Here's how the part is built. I have some questions about the finished solid (model axes, mm). A direction names the side the tool comes from. Give positions to 0.01 mm unless a question says otherwise; leave off trailing zeros. Write each loop counter-clockwise with the first axis right and the second up, starting at its lowest first coordinate (ties: lowest second). Pieces come first, ordered by that corner, then holes. Notation, with made-up numbers: (41, -9.5) - (70, -9.5) arc R25 cw to (70, 11.5) - close; hole circle Ø6 at (14.5, 14.25). An arc over 180 degrees is marked (long way). One line per item, written item: value. Start each with the question number.
1) Please list where these lines run through material, in increasing order: L1, parallel to X at y = 1.45, z = 7.4; L2, parallel to X at y = 3.6, z = -4; L3, parallel to Z at x = 3, y = 0.55. Write a range as [from, to].
2) I'm going to push flat-ended pins straight in: P1, Ø3, axis at x = -17.9, z = -5.4, coming from the +Y side; P2, Ø1.8, axis at x = -13, z = 41.02, coming from the +Y side. Where does each tip first touch, or does it pass through?
3) We'd pull the mould along Z, two halves only. Please class faces 4 (the flat face through (0, 0, 12)), 5 (the cylindrical face through (24.42, 2.46, -15.66)), 6 (the flat face through (-18, 2.5, 1)): +Z half, -Z half, draft (parallel to the pull), parting line (faces both ways), or undercut.
4) Imagine slicing it at D-D on x = -13. Write out the boundary of the cut face in (y, z).
5) On a 3-axis mill with a long thin cutter (end or side, diameter ignored), from which of +Z, -Z, +X, -X, +Y, -Y can I reach the whole of each face in a straight line? I mean faces 1 (the flat face through (15.8, 1, 1)), 2 (the flat face through (-29, 2, 12)), 3 (the flat face through (0, 3, -7.5)). Say none if no direction works.
6) Imagine slicing it at B-B on x = 13. Write out the boundary of the cut face in (y, z).
7) Imagine slicing it at C-C on x = -1. Write out the boundary of the cut face in (y, z), plus the area to 3 significant figures.
8) Imagine slicing it at A-A on z = 7.4. Write out the boundary of the cut face in (x, y).
from build123d import *

# Parameters (mm, degrees)
SKETCH1_R           = 1.45
SKETCH1_R_2         = 2
BOSS_EXTRUDE1_DEPTH = 5
SKETCH4_R           = 1.5
CUT_EXTRUDE2_DEPTH  = 5
SKETCH5_4_R         = 7.45
CUT_EXTRUDE6_DEPTH  = 5
SKETCH6_W           = 31.6
SKETCH6_H           = 17
SKETCH6_R           = 1.25
CUT_EXTRUDE8_DEPTH  = 5
SKETCH6_4_W         = 4.2
SKETCH6_4_H         = 4.2
SKETCH6_4_R         = 1.25
SKETCH6_4_H_2       = 8.6
CUT_EXTRUDE9_DEPTH  = 2.5


with BuildPart() as part:
    # Sketch1 → Boss-Extrude1 (new body)
    with BuildSketch(Plane(origin=(0, 0, 0), x_dir=(1, 0, 0), z_dir=(0, 1, 0))):
        with BuildLine():
            Line((-29, -28.777515286), (-29, 4.777515286))
            ThreePointArc((-29, 4.777515286), (-24.541437454, 15.541437454), (-13.777515286, 20))
            Line((-13.777515286, 20), (13.777515286, 20))
            ThreePointArc((13.777515286, 20), (24.541437454, 15.541437454), (29, 4.777515286))
            Line((29, 4.777515286), (29, -28.777515286))
            ThreePointArc((29, -28.777515286), (24.541437454, -39.541437454), (13.777515286, -44))
            Line((13.777515286, -44), (-13.777515286, -44))
            ThreePointArc((-13.777515286, -44), (-24.541437454, -39.541437454), (-29, -28.777515286))
        make_face()
        with Locations(Location((5.323230148, -16.145068002, 0), (0, 0, 270))):
            Circle(SKETCH1_R, mode=Mode.SUBTRACT)
        with Locations(Location((-9.753243024, -24, 0), (0, 0, 270))):
            Circle(SKETCH1_R_2, mode=Mode.SUBTRACT)
    extrude(amount=BOSS_EXTRUDE1_DEPTH)

    # Sketch4 → Cut-Extrude2 (cut)
    with BuildSketch(Plane(origin=(0, 5, 0), x_dir=(1, 0, 0), z_dir=(0, 1, 0))):
        with Locations(Location((13, 17.024816986, 0), (0, 0, 270))):
            Circle(SKETCH4_R)
        with Locations(Location((-13, 17.024816986, 0), (0, 0, 270))):
            Circle(SKETCH4_R)
        with Locations(Location((-13, -41.024816986, 0), (0, 0, 270))):
            Circle(SKETCH4_R)
        with Locations(Location((13, -41.024816986, 0), (0, 0, 270))):
            Circle(SKETCH4_R)
    extrude(amount=-CUT_EXTRUDE2_DEPTH, mode=Mode.SUBTRACT)

    # Sketch5<4> → Cut-Extrude6 (cut)
    with BuildSketch(Plane(origin=(0, 0, 0), x_dir=(1, 0, 0), z_dir=(0, 1, 0))):
        with Locations(Location((-9.753243024, -24, 0), (0, 0, 270))):
            Circle(SKETCH5_4_R)
    extrude(amount=CUT_EXTRUDE6_DEPTH, mode=Mode.SUBTRACT)

    # Sketch6 → Cut-Extrude8 (cut)
    with BuildSketch(Plane(origin=(0, 5, 0), x_dir=(1, 0, 0), z_dir=(0, 1, 0))):
        with Locations((0, -1)):
            Rectangle(SKETCH6_W, SKETCH6_H)
        with Locations(Location((-17.9, 5.4, 0), (0, 0, 270))):
            Circle(SKETCH6_R)
        with Locations(Location((-17.9, -7.4, 0), (0, 0, 270))):
            Circle(SKETCH6_R)
        with Locations(Location((17.9, 5.4, 0), (0, 0, 270))):
            Circle(SKETCH6_R)
        with Locations(Location((17.9, -7.4, 0), (0, 0, 270))):
            Circle(SKETCH6_R)
    extrude(amount=-CUT_EXTRUDE8_DEPTH, mode=Mode.SUBTRACT)

    # Sketch6<4> → Cut-Extrude9 (cut)
    # profile 1 of 6: a face of its own
    with BuildSketch(Plane(origin=(0, 5, 0), x_dir=(1, 0, 0), z_dir=(0, 1, 0))):
        with Locations((-17.9, 5.4)):
            Rectangle(SKETCH6_4_W, SKETCH6_4_H)
        with Locations(Location((-17.9, 5.4, 0), (0, 0, 270))):
            Circle(SKETCH6_4_R, mode=Mode.SUBTRACT)
    # profile 2 of 6: a face of its own
    with BuildSketch(Plane(origin=(0, 5, 0), x_dir=(1, 0, 0), z_dir=(0, 1, 0))):
        with Locations((17.9, 5.4)):
            Rectangle(SKETCH6_4_W, SKETCH6_4_H)
        with Locations(Location((17.9, 5.4, 0), (0, 0, 270))):
            Circle(SKETCH6_4_R, mode=Mode.SUBTRACT)
    # profile 3 of 6: a face of its own
    with BuildSketch(Plane(origin=(0, 5, 0), x_dir=(1, 0, 0), z_dir=(0, 1, 0))):
        with Locations((-17.9, -7.4)):
            Rectangle(SKETCH6_4_W, SKETCH6_4_H)
        with Locations(Location((-17.9, -7.4, 0), (0, 0, 270))):
            Circle(SKETCH6_4_R, mode=Mode.SUBTRACT)
    # profile 4 of 6: a face of its own
    with BuildSketch(Plane(origin=(0, 5, 0), x_dir=(1, 0, 0), z_dir=(0, 1, 0))):
        with Locations((17.9, -7.4)):
            Rectangle(SKETCH6_4_W, SKETCH6_4_H)
        with Locations(Location((17.9, -7.4, 0), (0, 0, 270))):
            Circle(SKETCH6_4_R, mode=Mode.SUBTRACT)
    # profile 5 of 6: a face of its own
    with BuildSketch(Plane(origin=(0, 5, 0), x_dir=(1, 0, 0), z_dir=(0, 1, 0))):
        with Locations((-17.9, -1)):
            Rectangle(SKETCH6_4_W, SKETCH6_4_H_2)
    # profile 6 of 6: a face of its own
    with BuildSketch(Plane(origin=(0, 5, 0), x_dir=(1, 0, 0), z_dir=(0, 1, 0))):
        with Locations((17.9, -1)):
            Rectangle(SKETCH6_4_W, SKETCH6_4_H_2)
    extrude(amount=-CUT_EXTRUDE9_DEPTH, mode=Mode.SUBTRACT)


solid = part.part
Numbers:
1. L1: [-29, -19.15], [-16.65, -15.8], [15.8, 16.65], [19.15, 29]
1. L2: [-29, -20], [20, 29]
1. L3: [-20, -7.5], [9.5, 44]
2. P1: y = 2.5
2. P2: through
3. face 4: draft
3. face 5: -Z half
3. face 6: undercut
4. outline: (0, -20) - (5, -20) - (5, -18.52) - (0, -18.52) - close; (0, -15.52) - (5, -15.52) - (5, -7.5) - (0, -7.5) - close; (0, 9.5) - (5, 9.5) - (5, 17.29) - (0, 17.29) - close; (0, 30.71) - (5, 30.71) - (5, 39.52) - (0, 39.52) - close; (0, 42.52) - (5, 42.52) - (5, 44) - (0, 44) - close
5. face 1: +Y, -Y
5. face 2: +Z, -Z, -X, +Y, -Y
5. face 3: +Y
6. outline: (0, -20) - (5, -20) - (5, -18.52) - (0, -18.52) - close; (0, -15.52) - (5, -15.52) - (5, -7.5) - (0, -7.5) - close; (0, 9.5) - (5, 9.5) - (5, 39.52) - (0, 39.52) - close; (0, 42.52) - (5, 42.52) - (5, 44) - (0, 44) - close
7. outline: (0, -20) - (5, -20) - (5, -7.5) - (0, -7.5) - close; (0, 9.5) - (5, 9.5) - (5, 44) - (0, 44) - close
7. area: 235 mm^2
8. outline: (-29, 0) - (-19.15, 0) - (-19.15, 2.5) - (-20, 2.5) - (-20, 5) - (-29, 5) - close; (-16.65, 0) - (-15.8, 0) - (-15.8, 2.5) - (-16.65, 2.5) - close; (15.8, 0) - (16.65, 0) - (16.65, 2.5) - (15.8, 2.5) - close; (19.15, 0) - (29, 0) - (29, 5) - (20, 5) - (20, 2.5) - (19.15, 2.5) - close
